```python
from build123d import *

# Parameters (mm, degrees)
SKETCH1_W           = 90
SKETCH1_H           = 70
BOSS_EXTRUDE1_DEPTH = 4
SKETCH2_R           = 1.75
CUT_EXTRUDE1_DEPTH  = 5
CHAMFER1_SIZE       = 2
CHAMFER2_SIZE       = 2
CHAMFER3_SIZE       = 2
CHAMFER4_SIZE       = 2
SKETCH5_W           = 70
SKETCH5_H           = 4
BOSS_EXTRUDE3_DEPTH = 10
SKETCH4_W           = 70
SKETCH4_H           = 4
BOSS_EXTRUDE4_DEPTH = 10
SKETCH6_R           = 1.75
CUT_EXTRUDE2_DEPTH  = 10
CHAMFER5_SIZE       = 2


with BuildPart() as part:
    # Sketch1 → Boss-Extrude1 (new body)
    with BuildSketch(Plane.XY):
        with Locations((44.768273235, 35.193370166)):
            Rectangle(SKETCH1_W, SKETCH1_H)
    extrude(amount=BOSS_EXTRUDE1_DEPTH)

    # Sketch2 → Cut-Extrude1 (cut)
    with BuildSketch(Plane.XY.offset(4)):
        with Locations((3.703568783, 2.693370166)):
            Circle(SKETCH2_R)
        with Locations((86.703568783, 2.694436567)):
            Circle(SKETCH2_R)
        with Locations((86.703273235, 67.693370166)):
            Circle(SKETCH2_R)
        with Locations((3.703273235, 67.693370166)):
            Circle(SKETCH2_R)
        with Locations((23.297725672, 13.693370166)):
            Circle(SKETCH2_R)
        with Locations((66.284051901, 13.693370166)):
            Circle(SKETCH2_R)
        with Locations((66.268273235, 56.693370166)):
            Circle(SKETCH2_R)
        with Locations((23.268273235, 56.693370166)):
            Circle(SKETCH2_R)
    extrude(amount=-CUT_EXTRUDE1_DEPTH, mode=Mode.SUBTRACT)

    # Chamfer1
    chamfer1_edges = [part.edges().sort_by_distance(p)[0] for p in [
        (89.768273235, 0.193370166, 2),
    ]]
    chamfer(chamfer1_edges, length=CHAMFER1_SIZE)

    # Chamfer2
    chamfer2_edges = [part.edges().sort_by_distance(p)[0] for p in [
        (-0.231726765, 0.193370166, 2),
    ]]
    chamfer(chamfer2_edges, length=CHAMFER2_SIZE)

    # Chamfer3
    chamfer3_edges = [part.edges().sort_by_distance(p)[0] for p in [
        (-0.231726765, 70.193370166, 2),
    ]]
    chamfer(chamfer3_edges, length=CHAMFER3_SIZE)

    # Chamfer4
    chamfer4_edges = [part.edges().sort_by_distance(p)[0] for p in [
        (89.768273235, 70.193370166, 2),
    ]]
    chamfer(chamfer4_edges, length=CHAMFER4_SIZE)

    # Sketch5 → Boss-Extrude3 (add)
    with BuildSketch(Plane(origin=(0, 70.193370166, 0), x_dir=(1, 0, 0), z_dir=(0, 1, 0))):
        with Locations((44.768273235, -2)):
            Rectangle(SKETCH5_W, SKETCH5_H)
    extrude(amount=BOSS_EXTRUDE3_DEPTH)

    # Sketch4 → Boss-Extrude4 (add)
    with BuildSketch(Plane(origin=(0, 0.193370166, 0), x_dir=(-1, 0, 0), z_dir=(0, -1, 0))):
        with Locations((-44.768273235, -2)):
            Rectangle(SKETCH4_W, SKETCH4_H)
    extrude(amount=BOSS_EXTRUDE4_DEPTH)

    # Sketch6 → Cut-Extrude2 (cut)
    with BuildSketch(Plane(origin=(0, 0, 0), x_dir=(-1, 0, 0), z_dir=(0, 0, -1))):
        with Locations((-12.268273235, 76.693370166)):
            Circle(SKETCH6_R)
        with Locations((-77.268273235, 76.693370166)):
            Circle(SKETCH6_R)
        with Locations((-77.268273235, -6.306629834)):
            Circle(SKETCH6_R)
        with Locations((-12.268273235, -6.306629834)):
            Circle(SKETCH6_R)
    extrude(amount=-CUT_EXTRUDE2_DEPTH, mode=Mode.SUBTRACT)

    # Chamfer5
    chamfer5_edges = [part.edges().sort_by_distance(p)[0] for p in [
        (9.768273235, 80.193370166, 2),
        (79.768273235, 80.193370166, 2),
        (9.768273235, -9.806629834, 2),
        (79.768273235, -9.806629834, 2),
    ]]
    chamfer(chamfer5_edges, length=CHAMFER5_SIZE)


solid = part.part
```
The model under review builds one solid part; all positions refer to its coordinate system, in mm. A direction names the side the tool comes from. Give positions to 0.01 mm unless a question says otherwise; leave off trailing zeros. Write each loop counter-clockwise with the first axis right and the second up, starting at its lowest first coordinate (ties: lowest second). Pieces come first, ordered by that corner, then holes.
(1) The part is to be moulded in two halves that separate along Y. For faces 5 (the cylindrical face through (88.373, 3.22, 2.028)), 6 (the flat face through (0.782, 69.207, 1.972)), 7 (the flat face through (-0.232, 35, 2)), say which applies: released by +Y, released by -Y, zero draft, split by the parting line, or undercut.
(2) To check wall thickness, follow L1, parallel to X at y = 57, z = 2.4; L2, parallel to Y at x = 13, z = 3.65; L3, parallel to X at y = 13, z = 3.15. State the ranges of each line that lie inside material, in increasing order.
(3) For P1, Ø3, axis at x = 77.27, y = -6.31, coming from the -Z side; P2, Ø1.2, axis at y = -5.5, z = 2, coming from the -X side, all flat-tipped, find the tip position at first contact; note any pin that passes through.
(4) Tool access review of faces 1 (the flat face through (84, 0.193, 2)), 2 (the flat face through (9.768, 74, 2)), 3 (the flat face through (9.768, -4, 2)), 4 (the flat face through (79.768, 74, 2)): name each direction out of +Z, -Z, +X, -X, +Y, -Y from which nothing blocks a thin tool from reaching the whole face with its end or side.
(5) Consider section B-B, the plane y = -3. Give the boundary of the cut face in (x, z), and give its area (3 significant figures).
(6) Consider section C-C, the plane x = 83.5. Give the boundary of the cut face in (y, z).
(7) Consider section A-A, the plane z = 2.5. Give the number of separate pieces and of enclosed holes in the cut face, and give its area (3 significant figures).
Returned:
1. face 5: undercut
1. face 6: released by +Y
1. face 7: zero draft
2. L1: x = -0.23 to 21.55, 24.99 to 64.55, 67.99 to 89.77
2. L2: y = -9.81 to -7.9, -4.72 to 75.1, 78.28 to 80.19
2. L3: x = -0.23 to 21.69, 24.9 to 64.68, 67.89 to 89.77
3. P1: passes through
3. P2: stops at x = 9.77
4. face 1: +Z, -Z, +X, -Y
4. face 2: +Z, -Z, -X, +Y
4. face 3: +Z, -Z, -X, -Y
4. face 4: +Z, -Z, +X, +Y
5. outline: (9.77, 0) - (79.77, 0) - (79.77, 4) - (9.77, 4) - close
5. area: 280 mm2
6. outline: (0.19, 0) - (70.19, 0) - (70.19, 4) - (0.19, 4) - close
7. separate pieces: 1
7. enclosed holes: 12
7. area: 7,570 mm2
